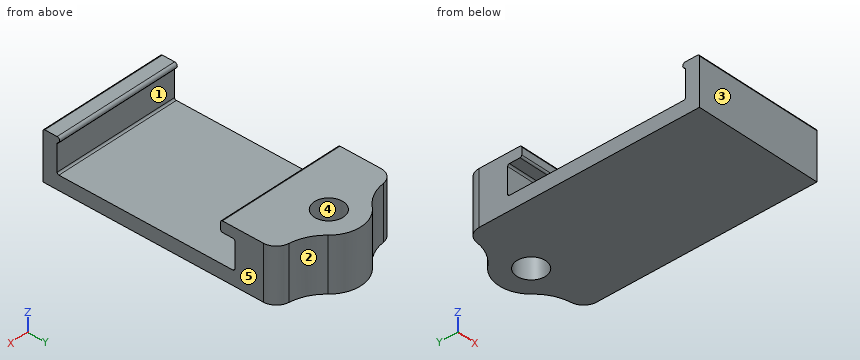
from build123d import *

# Parameters (mm, degrees)
BOSS_EXTRUDE1_DEPTH     = 14.2875
SKETCH3_W               = 28.575
SKETCH3_H               = 12.05625
BOSS_EXTRUDE2_DEPTH     = 12.7
SKETCH4_R               = 3.2385
CUT_EXTRUDE1_DEPTH      = 13.05625
FILLET1_R               = 0.396875
CUT_EXTRUDE2_DEPTH      = 1
CUT_EXTRUDE2_DEPTH_BACK = 13.05625
FILLET2_R               = 9.525
FILLET3_R               = 3.175


with BuildPart() as part:
    # Sketch2 → Boss-Extrude1 (new body, symmetric)
    with BuildSketch(Plane(origin=(0, 0, 0), x_dir=(0, 0, -1), z_dir=(1, 0, 0))):
        with BuildLine():
            Line((-3.25, 16.825), (-5.63125, 16.825))
            Line((-5.63125, 16.825), (-5.63125, 23.175))
            Line((-5.63125, 23.175), (6.425, 23.175))
            Line((6.425, 23.175), (6.425, -23.175))
            Line((6.425, -23.175), (-4.440625, -23.175))
            Line((-4.440625, -23.175), (-4.440625, -20))
            ThreePointArc((-4.440625, -20), (-3.8453125, -19.4046875), (-3.25, -20))
            Line((-3.25, -20), (3.25, -20))
            Line((3.25, -20), (3.25, 20))
            Line((3.25, 20), (-3.25, 20))
            Line((-3.25, 20), (-3.25, 16.825))
        make_face()
    extrude(amount=BOSS_EXTRUDE1_DEPTH, both=True)

    # Sketch3 → Boss-Extrude2 (add)
    with BuildSketch(Plane(origin=(0, 23.175, 0), x_dir=(1, 0, 0), z_dir=(0, 1, 0))):
        with Locations((0, 0.396875)):
            Rectangle(SKETCH3_W, SKETCH3_H)
    extrude(amount=BOSS_EXTRUDE2_DEPTH)

    # Sketch4 → Cut-Extrude1 (cut, through all)
    with BuildSketch(Plane.XY.offset(5.63125)):
        with Locations((0, 27.9375)):
            Circle(SKETCH4_R)
    extrude(amount=-CUT_EXTRUDE1_DEPTH, mode=Mode.SUBTRACT)

    # Fillet1
    fillet1_edges = [part.edges().sort_by_distance(p)[0] for p in [
        (0, 20, -3.25),
        (0, 20, 3.25),
        (0, 16.825, 3.25),
        (0, 16.825, 5.63125),
        (0, -23.175, 4.440625),
        (0, -20, 3.25),
        (0, -20, -3.25),
    ]]
    fillet(fillet1_edges, radius=FILLET1_R)

    # Sketch6 → Cut-Extrude2 (cut, two sides)
    with BuildSketch(Plane.XY.offset(5.63125)) as cut_extrude2_sk:
        with BuildLine():
            Line((-14.2875, 29.525), (-7.030241554, 29.525))
            ThreePointArc((-7.030241554, 29.525), (0, 35.14475), (7.030241554, 29.525))
            Line((7.030241554, 29.525), (14.2875, 29.525))
            Line((14.2875, 29.525), (14.2875, 35.875))
            Line((14.2875, 35.875), (-14.2875, 35.875))
            Line((-14.2875, 35.875), (-14.2875, 29.525))
        make_face()
    extrude(amount=CUT_EXTRUDE2_DEPTH, mode=Mode.SUBTRACT)
    extrude(cut_extrude2_sk.sketch, amount=-CUT_EXTRUDE2_DEPTH_BACK, mode=Mode.SUBTRACT)

    # Fillet2
    fillet2_edges = [part.edges().sort_by_distance(p)[0] for p in [
        (7.030241554, 29.525, -0.396875),
        (-7.030241554, 29.525, -0.396875),
    ]]
    fillet(fillet2_edges, radius=FILLET2_R)

    # Fillet3
    fillet3_edges = [part.edges().sort_by_distance(p)[0] for p in [
        (14.2875, 29.525, -0.396875),
        (-14.2875, 29.525, -0.396875),
    ]]
    fillet(fillet3_edges, radius=FILLET3_R)


solid = part.part
Read the model definition and answer for the solid it produces. Units are mm, in the model's axes. Face numbers are marked on the shaded views. A direction names the side the tool comes from. Round coordinates to 2 decimals unless told otherwise and drop trailing zeros. Write each loop counter-clockwise with the first axis right and the second up, starting at its lowest first coordinate (ties: lowest second). Pieces come first, ordered by that corner, then holes. Notation, with made-up numbers: (27.25, 36) - (64.25, 36) arc R14 cw to (64.25, 56) - close; hole circle Ø10 at (30.5, 27.25). An arc over 180 degrees is marked (long way). One line per question, with ' | ' between items. Start each with the question number.
1. Each of these flat-tipped pins is pushed along its axis until it touches: pin 1 (3 mm diameter, centred on x = 7, z = -1, fed in from +Y); pin 2 (0.8 mm diameter, centred on x = -4.5, y = -21, fed in from +Z); pin 3 (4 mm diameter, centred on x = -4, z = -5, fed in from +Y); pin 4 (1 mm diameter, centred on y = -3.5, z = -1, fed in from +X). Where does it stop, or does it pass through?
2. Find the intervals of material crossed by probe 1 along Y at (x, z) = (0, -1.25) (3 decimals); probe 2 along Y at (x, z) = (1.5, 2.75) (3 decimals); probe 3 along Z at (x, y) = (4.75, -16) (3 decimals), in increasing order. Write a range as [from, to].
3. Section A-A (x = 0) is taken. Determine the outline of the cut face in (y, z) (3 decimals).
4. Section B-B (x = -10.25) is taken. Determine the outline of the cut face in (y, z) (3 decimals).
5. For a pull along X with two mould halves and no side action, classify the marked faces 3, 4 and 5 as +X half, -X half, draft (parallel to the pull), parting line (faces both ways), or undercut.
6. For the marked faces 1 and 2, determine the directions among +Z, -Z, +X, -X, +Y, -Y from which every point of the face is accessible in a straight line to the end or side of a thin tool.
Filled in:
1) pin 1: y = 32.6 | pin 2: z = 4.44 | pin 3: y = 34.86 | pin 4: through
2) probe 1: [-23.175, -20], [20, 24.699], [31.176, 35.145] | probe 2: [-23.175, -20], [20, 25.067], [30.808, 34.987] | probe 3: [-6.425, -3.25]
3) outline: (-23.175, -6.425) - (24.699, -6.425) - (24.699, 5.631) - (17.222, 5.631) arc R0.397 ccw to (16.825, 5.234) - (16.825, 3.647) arc R0.397 ccw to (17.222, 3.25) - (19.603, 3.25) arc R0.397 cw to (20, 2.853) - (20, -2.853) arc R0.397 cw to (19.603, -3.25) - (-19.603, -3.25) arc R0.397 cw to (-20, -2.853) - (-20, 2.936) arc R0.397 cw to (-19.762, 3.3) arc R0.595 ccw to (-20, 4.441) - (-22.778, 4.441) arc R0.397 ccw to (-23.175, 4.044) - close; (31.176, -6.425) - (35.145, -6.425) - (35.145, 5.631) - (31.176, 5.631) - close
4) outline: (-23.175, -6.425) - (29.797, -6.425) - (29.797, 5.631) - (17.222, 5.631) arc R0.397 ccw to (16.825, 5.234) - (16.825, 3.647) arc R0.397 ccw to (17.222, 3.25) - (19.603, 3.25) arc R0.397 cw to (20, 2.853) - (20, -2.853) arc R0.397 cw to (19.603, -3.25) - (-19.603, -3.25) arc R0.397 cw to (-20, -2.853) - (-20, 2.936) arc R0.397 cw to (-19.762, 3.3) arc R0.595 ccw to (-20, 4.441) - (-22.778, 4.441) arc R0.397 ccw to (-23.175, 4.044) - close
5) face 3: draft | face 4: undercut | face 5: +X half
6) face 1: +X, -X | face 2: +Z, -Z, +X, +Y
